Can you work these out from the drawing? Everything is in mm from the part's minimum corner. A direction names the side the tool comes from. Round coordinates to 2 decimals unless told otherwise and drop trailing zeros. Loops run counter-clockwise (first coordinate to the right, second up) from the corner with the lowest first, then second, coordinate; pieces in that order, holes last. Notation, with made-up numbers: (89, -16.5) - (143, -16.5) arc R31 ccw to (143, 8.5) - close; hole circle Ø4 at (-36.75, 25). An arc over 180 degrees is marked (long way). Answer as a JSON object with one key per item and string values. Group by question number.
1) If we mould it in two halves opening along Z, with no side actions, what happens to the marked faces 1 and 2? For each: pulls with the +Z half, pulls with the -Z half, needs draft (parallel to the pull), parting line crosses it, or undercut.
2) Will these pins go through, and if not, where does the flat tip stop? P1, Ø5, axis at x = 9.5, z = 55.5, coming from the -Y side; P2, Ø6.5, axis at x = 4, z = 41, coming from the +Y side; P3, Ø1.6, axis at x = 15, z = 75, coming from the +Y side; P4, Ø0.6, axis at y = 0.5, z = 42, coming from the -X side.
3) I want a section at D-D, the plane y = 0.85. Please give me the cut outline in (x, z), then the cut area to 3 significant figures.
4) Which directions (+Z, -Z, +X, -X, +Y, -Y) give clear straight access to the entire face, cutting with the end or side of a thin tool? Please do the marked faces 3 and 4.
5) If I drill on line 1 along X through (y, z) = (2.6, 5); line 2 along X through (y, z) = (2.9, 25); line 3 along Y through (x, z) = (9.5, 60.5), over which ranges is the centre line in solid material (lowest first)? Write a range as [from, to].
6) I want a section at C-C, the plane z = 40. Please give me the cut outline in (x, y), then the cut area to 3 significant figures.
7) I want a section at A-A, the plane z = 25. Please give me the cut outline in (x, y), then the cut area to 3 significant figures.
8) I want a section at B-B, the plane x = 5. Please give me the cut outline in (y, z), then the cut area to 3 significant figures.
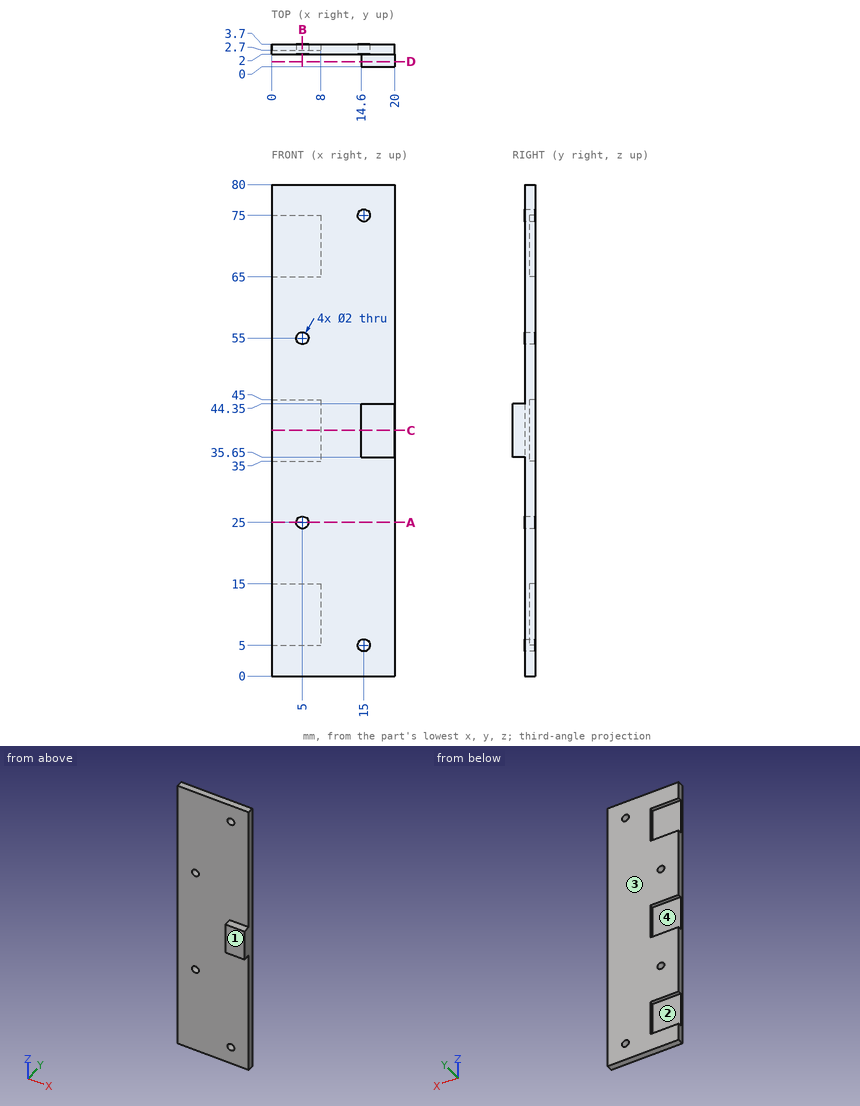
Outcome:
{
 "1": {"face 1": "needs draft", "face 2": "undercut"},
 "2": {"P1": "y = 2", "P2": "y = 2.7", "P3": "through", "P4": "x = 14.6"},
 "3": {"outline": "(14.6, 35.65) - (20, 35.65) - (20, 44.35) - (14.6, 44.35) - close", "area": "47.0 mm^2"},
 "4": {"face 3": "+Z, -Z, +X, -X, +Y", "face 4": "-X, +Y"},
 "5": {"line 1": "[0, 14], [16, 20]", "line 2": "[0, 4], [6, 20]", "line 3": "[2, 3.7]"},
 "6": {"outline": "(0, 2) - (14.6, 2) - (14.6, 0) - (20, 0) - (20, 3.7) - (8, 3.7) - (8, 2.7) - (0, 2.7) - close", "area": "36.8 mm^2"},
 "7": {"outline": "(0, 2) - (4, 2) - (4, 3.7) - (0, 3.7) - close; (6, 2) - (20, 2) - (20, 3.7) - (6, 3.7) - close", "area": "30.6 mm^2"},
 "8": {"outline": "(2, 0) - (3.7, 0) - (3.7, 5) - (2.7, 5) - (2.7, 15) - (3.7, 15) - (3.7, 24) - (2, 24) - close; (2, 26) - (3.7, 26) - (3.7, 35) - (2.7, 35) - (2.7, 45) - (3.7, 45) - (3.7, 54) - (2, 54) - close; (2, 56) - (3.7, 56) - (3.7, 65) - (2.7, 65) - (2.7, 75) - (3.7, 75) - (3.7, 80) - (2, 80) - close", "area": "99.2 mm^2"}
}
